Here's how the part is built. I have some questions about the finished solid (model axes, mm). Face numbers are marked on the shaded views. A direction names the side the tool comes from. Coordinates: 2 decimals unless noted, no trailing zeros. Write each loop counter-clockwise with the first axis right and the second up, starting at its lowest first coordinate (ties: lowest second). Pieces come first, ordered by that corner, then holes. Notation, with made-up numbers: M 83.5,4 L 129.5,4 A12 cw 129.5,15 Z; hole C -17,26 d4. An arc over 180 degrees is marked long. Use a Markdown table: item, result.
```python
from build123d import *

# Parameters (mm, degrees)
SKETCH_1_R      = 1.55
EXTRUDE_1_DEPTH = 5


with BuildPart() as part:
    # 草圖1 → 填料-伸長1 (new body)
    with BuildSketch(Plane.XY):
        with BuildLine():
            Line((-4.5, 1), (-3.354101966, 1))
            ThreePointArc((-3.354101966, 1), (0, 3.5), (3.354101966, 1))
            Line((3.354101966, 1), (4.5, 1))
            Line((4.5, 1), (4.5, -1))
            Line((4.5, -1), (3.354101966, -1))
            ThreePointArc((3.354101966, -1), (0, -3.5), (-3.354101966, -1))
            Line((-3.354101966, -1), (-4.5, -1))
            Line((-4.5, -1), (-4.5, 1))
        make_face()
        Circle(SKETCH_1_R, mode=Mode.SUBTRACT)
    extrude(amount=EXTRUDE_1_DEPTH)


solid = part.part
```
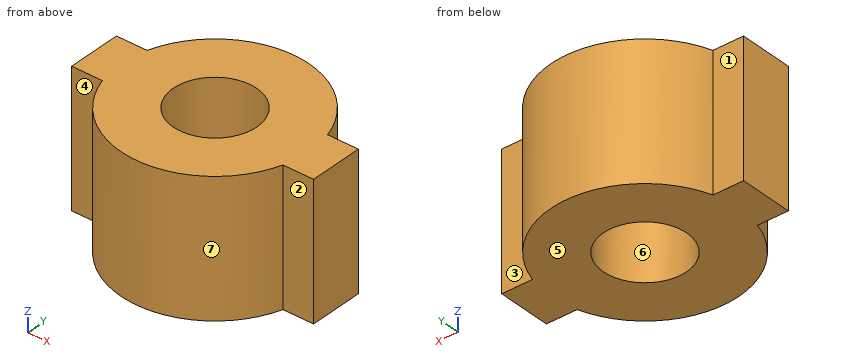
1. Will these pins go through, and if not, where does the flat tip stop? pin 1 Ø1.5 at (x, z) = (1, 2.5) entering from +Y; pin 2 Ø0.6 at (x, z) = (4, 2.5) entering from -Y.
Answers follow:
| item | result |
|---|---|
| pin 1 | stops at y = 3.49 |
| pin 2 | stops at y = -1 |
2. Which directions (+Z, -Z, +X, -X, +Y, -Y) give clear straight access to the entire face, cutting with the end or side of a thin tool? Please do the marked faces 1, 2, 3 and 4.
Answers follow:
| item | result |
|---|---|
| face 1 | +Z, -Z, -X, +Y |
| face 2 | +Z, -Z, +X, -Y |
| face 3 | +Z, -Z, +X, +Y |
| face 4 | +Z, -Z, -X, -Y |
3. We'd pull the mould along X, two halves only. Please class the marked faces 5, 6 and 7: +X half, -X half, draft (parallel to the pull), parting line (faces both ways), or undercut.
Answers follow:
| item | result |
|---|---|
| face 5 | draft |
| face 6 | undercut |
| face 7 | parting line |
4. Suppose I cut it at C-C on z = 2.1. Write out the boundary of the cut face in (x, y), and give its area (3 significant figures).
Answers follow:
| item | result |
|---|---|
| outline | M -4.5,-1 L -3.35,-1 A3.5 ccw 3.35,-1 L 4.5,-1 L 4.5,1 L 3.35,1 A3.5 ccw -3.35,1 L -4.5,1 Z; hole C 0,0 d3.1 |
| area | 35.1 mm2 |
5. Suppose I cut it at B-B on x = 0. Write out the boundary of the cut face in (y, z), and give its area (3 significant figures).
Answers follow:
| item | result |
|---|---|
| outline | M -3.5,0 L -1.55,0 L -1.55,5 L -3.5,5 Z; M 1.55,0 L 3.5,0 L 3.5,5 L 1.55,5 Z |
| area | 19.5 mm2 |
6. I need wall thicknesses on probe 1 along X at (y, z) = (-1.25, 1.9); probe 2 along X at (y, z) = (-2.5, 1.2); probe 3 along Y at (x, z) = (-3, 0.45). Which ranges of each line are inside material? Lowest first, please.
Answers follow:
| item | result |
|---|---|
| probe 1 | x = -3.27 to -0.92, 0.92 to 3.27 |
| probe 2 | x = -2.45 to 2.45 |
| probe 3 | y = -1.8 to 1.8 |
7. Suppose I cut it at D-D on x = 3.25. Write out the boundary of the cut face in (y, z).
Answers follow:
| item | result |
|---|---|
| outline | M -1.3,0 L 1.3,0 L 1.3,5 L -1.3,5 Z |
8. Suppose I cut it at A-A on y = 0. Write out the boundary of the cut face in (x, z).
Answers follow:
| item | result |
|---|---|
| outline | M -4.5,0 L -1.55,0 L -1.55,5 L -4.5,5 Z; M 1.55,0 L 4.5,0 L 4.5,5 L 1.55,5 Z |
